Geometry: final body of the model. Coordinates: model frame, mm. A direction names the side the tool comes from. Give positions to 0.01 mm unless a question says otherwise; leave off trailing zeros. Write each loop counter-clockwise with the first axis right and the second up, starting at its lowest first coordinate (ties: lowest second). Pieces come first, ordered by that corner, then holes. Notation, with made-up numbers: (46.5, -8) - (50.5, -8) arc R10 cw to (50.5, 10) - close; hole circle Ø8 at (33, -25.5). An arc over 180 degrees is marked (long way). One line per question, with ' | ' between items. Start each with the question number.
```python
from build123d import *

# Parameters (mm, degrees)
BOSS_EXTRUDE1_DEPTH = 6.096


with BuildPart() as part:
    # Sketch1 → Boss-Extrude1 (new body)
    with BuildSketch(Plane.XY):
        with BuildLine():
            Line((0, 0), (13, 0))
            add(Edge.make_bspline(
                [(20, 0), (20, 3), (16.5, 3), (13, 3), (13, 0)],
                knots=[3.141592654, 3.141592654, 3.141592654, 4.71238898, 4.71238898, 6.283185307, 6.283185307, 6.283185307], degree=2, weights=[1, 0.707106781, 1, 0.707106781, 1]))
            Line((20, 0), (223, 0))
            add(Edge.make_bspline(
                [(230, 0), (230, 3), (226.5, 3), (223, 3), (223, 0)],
                knots=[3.141592654, 3.141592654, 3.141592654, 4.71238898, 4.71238898, 6.283185307, 6.283185307, 6.283185307], degree=2, weights=[1, 0.707106781, 1, 0.707106781, 1]))
            Line((230, 0), (250, 0))
            Line((250, 0), (228.197731568, 15.697633271))
            Line((228.197731568, 15.697633271), (231.759653176, 20.644746617))
            Line((231.759653176, 20.644746617), (215.528966347, 32.330841134))
            Line((215.528966347, 32.330841134), (211.967044739, 27.383727788))
            Line((211.967044739, 27.383727788), (190.164776306, 43.081361059))
            Line((190.164776306, 43.081361059), (193.726697915, 48.028474405))
            Line((193.726697915, 48.028474405), (177.496011086, 59.714568922))
            Line((177.496011086, 59.714568922), (173.934089477, 54.767455576))
            Line((173.934089477, 54.767455576), (152.131821045, 70.465088847))
            Line((152.131821045, 70.465088847), (155.693742654, 75.412202193))
            Line((155.693742654, 75.412202193), (139.463055825, 87.09829671))
            Line((139.463055825, 87.09829671), (135.901134216, 82.151183364))
            Line((135.901134216, 82.151183364), (114.098865784, 97.848816636))
            Line((114.098865784, 97.848816636), (117.660787393, 102.795929981))
            Line((117.660787393, 102.795929981), (101.430100564, 114.482024498))
            Line((101.430100564, 114.482024498), (97.868178955, 109.534911153))
            Line((97.868178955, 109.534911153), (76.065910523, 125.232544424))
            Line((76.065910523, 125.232544424), (79.627832131, 130.179657769))
            Line((79.627832131, 130.179657769), (63.397145302, 141.865752286))
            Line((63.397145302, 141.865752286), (59.835223694, 136.918638941))
            Line((59.835223694, 136.918638941), (38.032955261, 152.616272212))
            Line((38.032955261, 152.616272212), (41.59487687, 157.563385557))
            Line((41.59487687, 157.563385557), (25.364190041, 169.249480074))
            Line((25.364190041, 169.249480074), (21.802268432, 164.302366729))
            Line((21.802268432, 164.302366729), (0, 180))
            Line((0, 180), (0, 0))
        make_face()
    extrude(amount=BOSS_EXTRUDE1_DEPTH)


solid = part.part
```
1) Line query: L1, parallel to X at y = 57.5, z = 0.5; L2, parallel to Y at x = 128, z = 1; L3, parallel to X at y = 13.5, z = 3. Output: solid intervals per line, ascending.
2) First-contact query: pin 1 Ø2 at (x, z) = (216.5, 3.5) entering from +Y; pin 2 Ø2 at (y, z) = (154, 3.5) entering from +X; pin 3 Ø4 at (x, y) = (134.5, 88) entering from -Z. Flat tips, straight axial feed; report the tip coordinate or a pass-through.
3) Reachability of faces 4 (the flat face through (39.79, 155.06, 3.01)), 5 (the flat face through (175.74, 57.276, 3.005)), 6 (the flat face through (120, 0, 3)) from +Z, -Z, +X, -X, +Y, -Y: full face, straight path, thin tool, end or side. Return the list, or none.
4) Section B-B, the plane y = 63. Output: boundary loops of the cut face in (x, z), plus the area to 3 significant figures.
5) Section A-A, the plane x = 92. Output: boundary loops of the cut face in (y, z).
6) Pull-direction query (Y, two-part tool) for faces 1 (the flat face through (77.82, 127.67, 3.01)), 2 (the flat face through (6, 0, 3)), 3 (the flat face through (61.641, 139.427, 3.005)); classes: +Y half, -Y half, draft (parallel to the pull), parting line (faces both ways), or undercut.
Answer key:
1) L1: 0 to 170.14, 175.9 to 180.57 | L2: 0 to 87.84 | L3: 0 to 231.25
2) pin 1: y = 32.33 | pin 2: x = 39.75 | pin 3: through
3) face 4: +Z, -Z, +X | face 5: +Z, -Z, +Y | face 6: +Z, -Z, +X, -X, -Y
4) outline: (0, 0) - (162.5, 0) - (162.5, 6.1) - (0, 6.1) - close | area: 991 mm^2
5) outline: (0, 0) - (113.76, 0) - (113.76, 6.1) - (0, 6.1) - close
6) face 1: undercut | face 2: -Y half | face 3: +Y half
